from build123d import *

# Parameters (mm, degrees)
F0_W         = 254
F0_H         = 203.2
F1_DEPTH     = 12.7
F4_DEPTH     = 254.001
F2_W         = 76.2
F2_H         = 12.7
F5_DEPTH     = 12.701
F6_T1_DEPTH  = 228.6
F6_T3_DEPTH  = 279.4
F6_T5_DEPTH  = 76.2
F6_T7_DEPTH  = 25.4
F6_T9_DEPTH  = 152.4
F6_T11_DEPTH = 76.2
F6_T17_DEPTH = 38.1
F6_T21_DEPTH = 165.1
F6_T28_DEPTH = 38.1
F6_T32_DEPTH = 165.1
F6_T39_DEPTH = 38.1
F6_T43_DEPTH = 165.1
F6_T50_DEPTH = 165.1
F6_T54_DEPTH = 38.1
F7_T1_DEPTH  = 12.7000000002
F7_T4_ANGLE  = 90
F7_T6_ANGLE  = 90
F7_T8_ANGLE  = 90
F7_T10_ANGLE = 90


# Not quite as in the source:
# - a fillet or chamfer that OpenCascade refuses, or shapes differently, is made with other operations: its cross-section is extruded or revolved along the edge and cut away or added


with BuildPart() as f1:
    # F0 (on Top) → F1 (new body)
    with BuildSketch(Plane.XY):
        Rectangle(F0_W, F0_H)
    extrude(amount=F1_DEPTH)

    # F3 (on face) → F4 (cut, through all)
    with BuildSketch(Plane(origin=(-127, 0, 0), x_dir=(0, -1, 0), z_dir=(-1, 0, 0))):
        with BuildLine():
            ThreePointArc((-92.075, 6.35), (-95.25, 9.525), (-98.425, 6.35))
            Line((-98.425, 6.35), (-92.075, 6.35))
        make_face()
        with BuildLine():
            Line((-92.075, 6.35), (-98.425, 6.35))
            ThreePointArc((-98.425, 6.35), (-95.25, 3.175), (-92.075, 6.35))
        make_face()
    extrude(amount=-F4_DEPTH, mode=Mode.SUBTRACT)

    # F2 (on face) → F5 (cut, through all)
    with BuildSketch(Plane.XY.offset(12.7)):
        with Locations((-38.1, 95.25)):
            Rectangle(F2_W, F2_H)
        with Locations((38.1, 95.25)):
            Rectangle(F2_W, F2_H)
    extrude(amount=-F5_DEPTH, mode=Mode.SUBTRACT)

    # F6: fillet of radius 5.08 on 16 edges, made by hand

    # F6_s2 → F6_t1 (cut)
    with BuildSketch(Plane.XZ.offset(-114.3)):
        with BuildLine():
            ThreePointArc((121.92, 12.7), (125.5121024484, 11.2121024484), (127, 7.62))
            Line((127, 7.62), (127, 12.7))
            Line((127, 12.7), (121.92, 12.7))
        make_face()
        with BuildLine():
            ThreePointArc((-121.92, 12.7), (-125.5121024484, 11.2121024484), (-127, 7.62))
            Line((-127, 7.62), (-127, 12.7))
            Line((-127, 12.7), (-121.92, 12.7))
        make_face()
        with BuildLine():
            ThreePointArc((121.92, 0), (125.5121024484, 1.4878975516), (127, 5.08))
            Line((127, 5.08), (127, 0))
            Line((127, 0), (121.92, 0))
        make_face()
        with BuildLine():
            ThreePointArc((-121.92, 0), (-125.5121024484, 1.4878975516), (-127, 5.08))
            Line((-127, 5.08), (-127, 0))
            Line((-127, 0), (-121.92, 0))
        make_face()
    extrude(amount=F6_T1_DEPTH, mode=Mode.SUBTRACT)

    # F6_s4 → F6_t3 (cut)
    with BuildSketch(Plane.YZ.offset(-139.7)):
        with BuildLine():
            ThreePointArc((-96.52, 12.7), (-100.1121024484, 11.2121024484), (-101.6, 7.62))
            Line((-101.6, 7.62), (-101.6, 12.7))
            Line((-101.6, 12.7), (-96.52, 12.7))
        make_face()
        with BuildLine():
            ThreePointArc((-96.52, 0), (-100.1121024484, 1.4878975516), (-101.6, 5.08))
            Line((-101.6, 5.08), (-101.6, 0))
            Line((-101.6, 0), (-96.52, 0))
        make_face()
    extrude(amount=F6_T3_DEPTH, mode=Mode.SUBTRACT)

    # F6_s6 → F6_t5 (cut)
    with BuildSketch(Plane.YZ.offset(-139.7)):
        with BuildLine():
            ThreePointArc((96.52, 12.7), (100.1121024484, 11.2121024484), (101.6, 7.62))
            Line((101.6, 7.62), (101.6, 12.7))
            Line((101.6, 12.7), (96.52, 12.7))
        make_face()
        with BuildLine():
            ThreePointArc((96.52, 0), (100.1121024484, 1.4878975516), (101.6, 5.08))
            Line((101.6, 5.08), (101.6, 0))
            Line((101.6, 0), (96.52, 0))
        make_face()
    extrude(amount=F6_T5_DEPTH, mode=Mode.SUBTRACT)

    # F6_s8 → F6_t7 (cut)
    with BuildSketch(Plane.XZ.offset(-114.3)):
        with BuildLine():
            ThreePointArc((-81.28, 12.7), (-77.6878975516, 11.2121024484), (-76.2, 7.62))
            Line((-76.2, 7.62), (-76.2, 12.7))
            Line((-76.2, 12.7), (-81.28, 12.7))
        make_face()
        with BuildLine():
            ThreePointArc((76.2, 7.62), (77.6878975516, 11.2121024484), (81.28, 12.7))
            Line((81.28, 12.7), (76.2, 12.7))
            Line((76.2, 12.7), (76.2, 7.62))
        make_face()
        with BuildLine():
            ThreePointArc((-81.28, 0), (-77.6878975516, 1.4878975516), (-76.2, 5.08))
            Line((-76.2, 5.08), (-76.2, 0))
            Line((-76.2, 0), (-81.28, 0))
        make_face()
        with BuildLine():
            ThreePointArc((81.28, 0), (77.6878975516, 1.4878975516), (76.2, 5.08))
            Line((76.2, 5.08), (76.2, 0))
            Line((76.2, 0), (81.28, 0))
        make_face()
    extrude(amount=F6_T7_DEPTH, mode=Mode.SUBTRACT)

    # F6_s10 → F6_t9 (cut)
    with BuildSketch(Plane.YZ.offset(-76.2)):
        with BuildLine():
            ThreePointArc((83.82, 12.7), (87.4121024484, 11.2121024484), (88.9, 7.62))
            Line((88.9, 7.62), (88.9, 12.7))
            Line((88.9, 12.7), (83.82, 12.7))
        make_face()
        with BuildLine():
            ThreePointArc((83.82, 0), (87.4121024484, 1.4878975516), (88.9, 5.08))
            Line((88.9, 5.08), (88.9, 0))
            Line((88.9, 0), (83.82, 0))
        make_face()
    extrude(amount=F6_T9_DEPTH, mode=Mode.SUBTRACT)

    # F6_s12 → F6_t11 (cut)
    with BuildSketch(Plane.YZ.offset(63.5)):
        with BuildLine():
            ThreePointArc((101.6, 7.62), (100.1121024484, 11.2121024484), (96.52, 12.7))
            Line((96.52, 12.7), (101.6, 12.7))
            Line((101.6, 12.7), (101.6, 7.62))
        make_face()
        with BuildLine():
            ThreePointArc((101.6, 5.08), (100.1121024484, 1.4878975516), (96.52, 0))
            Line((96.52, 0), (101.6, 0))
            Line((101.6, 0), (101.6, 5.08))
        make_face()
    extrude(amount=F6_T11_DEPTH, mode=Mode.SUBTRACT)


with BuildPart() as f6_tool15:
    # F6_s16 → F6_t17 (new body)
    with BuildSketch(Plane.XZ.offset(-114.3)):
        with BuildLine():
            ThreePointArc((-81.28, 12.7), (-77.6878975516, 11.2121024484), (-76.2, 7.62))
            Line((-76.2, 7.62), (-76.2, 12.7))
            Line((-76.2, 12.7), (-81.28, 12.7))
        make_face()
    extrude(amount=F6_T17_DEPTH)

    split(bisect_by=Plane.XZ.offset(-88.9), keep=Keep.TOP)


with BuildPart() as f6_tool19:
    # F6_s20 → F6_t21 (new body)
    with BuildSketch(Plane.YZ.offset(-88.9)):
        with BuildLine():
            ThreePointArc((83.82, 12.7), (87.4121024484, 11.2121024484), (88.9, 7.62))
            Line((88.9, 7.62), (88.9, 12.7))
            Line((88.9, 12.7), (83.82, 12.7))
        make_face()
    extrude(amount=F6_T21_DEPTH)

    split(bisect_by=Plane.YZ.offset(-76.2), keep=Keep.BOTTOM)


with BuildPart() as f6_tool15_1:
    add(f6_tool15.part)

    # F6_t23: intersect F6_tool19
    add(f6_tool19.part, mode=Mode.INTERSECT)


with BuildPart() as f1_1:
    add(f1.part)

    # F6_t13: cut F6_tool15
    add(f6_tool15_1.part, mode=Mode.SUBTRACT)


with BuildPart() as f6_tool26:
    # F6_s27 → F6_t28 (new body)
    with BuildSketch(Plane.XZ.offset(-76.2)):
        with BuildLine():
            ThreePointArc((76.2, 7.62), (77.6878975516, 11.2121024484), (81.28, 12.7))
            Line((81.28, 12.7), (76.2, 12.7))
            Line((76.2, 12.7), (76.2, 7.62))
        make_face()
    extrude(amount=-F6_T28_DEPTH)

    split(bisect_by=Plane.XZ.offset(-88.9), keep=Keep.TOP)


with BuildPart() as f6_tool30:
    # F6_s31 → F6_t32 (new body)
    with BuildSketch(Plane.YZ.offset(-76.2)):
        with BuildLine():
            ThreePointArc((83.82, 12.7), (87.4121024484, 11.2121024484), (88.9, 7.62))
            Line((88.9, 7.62), (88.9, 12.7))
            Line((88.9, 12.7), (83.82, 12.7))
        make_face()
    extrude(amount=F6_T32_DEPTH)

    split(bisect_by=Plane.YZ.offset(76.2), keep=Keep.TOP)


with BuildPart() as f6_tool26_1:
    add(f6_tool26.part)

    # F6_t34: intersect F6_tool30
    add(f6_tool30.part, mode=Mode.INTERSECT)


with BuildPart() as f1_2:
    add(f1_1.part)

    # F6_t24: cut F6_tool26
    add(f6_tool26_1.part, mode=Mode.SUBTRACT)


with BuildPart() as f6_tool37:
    # F6_s38 → F6_t39 (new body)
    with BuildSketch(Plane.XZ.offset(-114.3)):
        with BuildLine():
            ThreePointArc((-81.28, 0), (-77.6878975516, 1.4878975516), (-76.2, 5.08))
            Line((-76.2, 5.08), (-76.2, 0))
            Line((-76.2, 0), (-81.28, 0))
        make_face()
    extrude(amount=F6_T39_DEPTH)

    split(bisect_by=Plane.XZ.offset(-88.9), keep=Keep.TOP)


with BuildPart() as f6_tool41:
    # F6_s42 → F6_t43 (new body)
    with BuildSketch(Plane.YZ.offset(-88.9)):
        with BuildLine():
            ThreePointArc((83.82, 0), (87.4121024484, 1.4878975516), (88.9, 5.08))
            Line((88.9, 5.08), (88.9, 0))
            Line((88.9, 0), (83.82, 0))
        make_face()
    extrude(amount=F6_T43_DEPTH)

    split(bisect_by=Plane.YZ.offset(-76.2), keep=Keep.BOTTOM)


with BuildPart() as f6_tool37_1:
    add(f6_tool37.part)

    # F6_t45: intersect F6_tool41
    add(f6_tool41.part, mode=Mode.INTERSECT)


with BuildPart() as f1_3:
    add(f1_2.part)

    # F6_t35: cut F6_tool37
    add(f6_tool37_1.part, mode=Mode.SUBTRACT)


with BuildPart() as f6_tool48:
    # F6_s49 → F6_t50 (new body)
    with BuildSketch(Plane.YZ.offset(-76.2)):
        with BuildLine():
            ThreePointArc((83.82, 0), (87.4121024484, 1.4878975516), (88.9, 5.08))
            Line((88.9, 5.08), (88.9, 0))
            Line((88.9, 0), (83.82, 0))
        make_face()
    extrude(amount=F6_T50_DEPTH)

    split(bisect_by=Plane.YZ.offset(76.2), keep=Keep.TOP)


with BuildPart() as f6_tool52:
    # F6_s53 → F6_t54 (new body)
    with BuildSketch(Plane.XZ.offset(-76.2)):
        with BuildLine():
            ThreePointArc((81.28, 0), (77.6878975516, 1.4878975516), (76.2, 5.08))
            Line((76.2, 5.08), (76.2, 0))
            Line((76.2, 0), (81.28, 0))
        make_face()
    extrude(amount=-F6_T54_DEPTH)

    split(bisect_by=Plane.XZ.offset(-88.9), keep=Keep.TOP)


with BuildPart() as f6_tool48_1:
    add(f6_tool48.part)

    # F6_t56: intersect F6_tool52
    add(f6_tool52.part, mode=Mode.INTERSECT)


with BuildPart() as f1_4:
    add(f1_3.part)

    # F6_t46: cut F6_tool48
    add(f6_tool48_1.part, mode=Mode.SUBTRACT)

    # F7: fillet of radius 12.7 on 2 edges, made by hand

    # F7_s2 → F7_t1 (cut)
    with BuildSketch(Plane.XY):
        with BuildLine():
            ThreePointArc((-114.3, -101.6), (-123.2802561211, -97.8802561211), (-127, -88.9))
            Line((-127, -88.9), (-127, -101.6))
            Line((-127, -101.6), (-114.3, -101.6))
        make_face()
        with BuildLine():
            ThreePointArc((114.3, -101.6), (123.2802561211, -97.8802561211), (127, -88.9))
            Line((127, -88.9), (127, -101.6))
            Line((127, -101.6), (114.3, -101.6))
        make_face()
    extrude(amount=F7_T1_DEPTH, mode=Mode.SUBTRACT)

    # F7_s3 → F7_t4 (revolve, cut)
    with BuildSketch(Plane.XZ.offset(88.9)):
        with BuildLine():
            ThreePointArc((121.9199999999, 0), (125.5121024484, 1.4878975516), (127, 5.0800000001))
            Line((127, 5.0800000001), (127, 0))
            Line((127, 0), (121.9199999999, 0))
        make_face()
    revolve(axis=Axis((114.3, -88.9, 0), (0, 0, -1)), revolution_arc=F7_T4_ANGLE, mode=Mode.SUBTRACT)

    # F7_s5 → F7_t6 (revolve, cut)
    with BuildSketch(Plane.YZ.offset(114.3)):
        with BuildLine():
            ThreePointArc((-96.5199999999, 12.7), (-100.1121024484, 11.2121024484), (-101.6, 7.6199999999))
            Line((-101.6, 7.6199999999), (-101.6, 12.7))
            Line((-101.6, 12.7), (-96.5199999999, 12.7))
        make_face()
    revolve(axis=Axis((114.3, -88.9, 12.7), (0, 0, 1)), revolution_arc=F7_T6_ANGLE, mode=Mode.SUBTRACT)

    # F7_s7 → F7_t8 (revolve, cut)
    with BuildSketch(Plane.YZ.offset(-114.3)):
        with BuildLine():
            ThreePointArc((-96.5199999999, 0), (-100.1121024484, 1.4878975516), (-101.6, 5.0800000001))
            Line((-101.6, 5.0800000001), (-101.6, 0))
            Line((-101.6, 0), (-96.5199999999, 0))
        make_face()
    revolve(axis=Axis((-114.3, -88.9, 0), (0, 0, -1)), revolution_arc=F7_T8_ANGLE, mode=Mode.SUBTRACT)

    # F7_s9 → F7_t10 (revolve, cut)
    with BuildSketch(Plane.XZ.offset(88.9)):
        with BuildLine():
            ThreePointArc((-121.9199999999, 12.7), (-125.5121024484, 11.2121024484), (-127, 7.6199999999))
            Line((-127, 7.6199999999), (-127, 12.7))
            Line((-127, 12.7), (-121.9199999999, 12.7))
        make_face()
    revolve(axis=Axis((-114.3, -88.9, 12.7), (0, 0, 1)), revolution_arc=F7_T10_ANGLE, mode=Mode.SUBTRACT)


solid = f1_4.part
Design review of the part built by this model. Coordinates are the model's own, in mm. A direction names the side the tool comes from. Give positions to 0.01 mm unless a question says otherwise; leave off trailing zeros. Write each loop counter-clockwise with the first axis right and the second up, starting at its lowest first coordinate (ties: lowest second). Pieces come first, ordered by that corner, then holes. Notation, with made-up numbers: M 35.5,45 L 45.5,45 A6 ccw 45.5,52 Z; hole C -19.5,63.5 d3. An arc over 180 degrees is marked long. Answer as a JSON object with one key per item and string values. Group by question number.
1) For line 1 along Z through (x, y) = (-97, 95.25) (3 decimals); line 2 along Y through (x, z) = (-52, 8); line 3 along X through (y, z) = (-45, 7.75), list the stretches that pass through material, from the lowest coordinate up.
2) Tool access review of faces 1 (the face through (-1.138, 87.372, 1.449)), 2 (the face through (77.649, 92.586, 11.172)), 3 (the face through (-101.96, 98.28, 5.4)): name each direction out of +Z, -Z, +X, -X, +Y, -Y from which nothing blocks a thin tool from reaching the whole face with its end or side.
3) We need section B-B (x = 33). Give the boundary of the cut face in (y, z).
4) Mouldability with a two-part tool opening along X and no side actions: class faces 4 (the face through (-101.956, 100.072, 11.251)), 5 (the face through (-125.472, 7.684, 11.251)), 6 (the face through (77.728, 92.586, 1.449)) as released by +X, released by -X, zero draft, split by the parting line, or undercut.
5) Clearance check with flat-ended pins moving along their axes: pin 1 Ø1.5 at (y, z) = (31.5, 11) entering from -X; pin 2 Ø3 at (x, z) = (-8.5, 6.5) entering from +Y; pin 3 Ø1 at (x, z) = (-42, 1.5) entering from +Y. State where each tip first meets the part, or that it passes through.
6) We need section A-A (x = 89.5). Give the boundary of the cut face in (y, z) (3 decimals), and give its area (3 significant figures).
Answer key:
{
 "1": {"line 1": "z = 0 to 3.175, 9.525 to 12.7", "line 2": "y = -101.59 to 88.89", "line 3": "x = -127 to 127"},
 "2": {"face 1": "-Z, +Y", "face 2": "+Z, +Y", "face 3": "+X, -X"},
 "3": {"outline": "M -101.6,5.08 A5.08 ccw -96.52,0 L 83.82,0 A5.08 ccw 88.9,5.08 L 88.9,7.62 A5.08 ccw 83.82,12.7 L -96.52,12.7 A5.08 ccw -101.6,7.62 Z"},
 "4": {"face 4": "zero draft", "face 5": "released by -X", "face 6": "undercut"},
 "5": {"pin 1": "stops at x = -126.27", "pin 2": "stops at y = 88.9", "pin 3": "stops at y = 87.86"},
 "6": {"outline": "M -101.6,5.08 A5.08 ccw -96.52,0 L 96.52,0 A5.08 ccw 101.6,5.08 L 101.6,7.62 A5.08 ccw 96.52,12.7 L -96.52,12.7 A5.08 ccw -101.6,7.62 Z; hole C 95.25,6.35 d6.35", "area": "2,530 mm²"}
}
